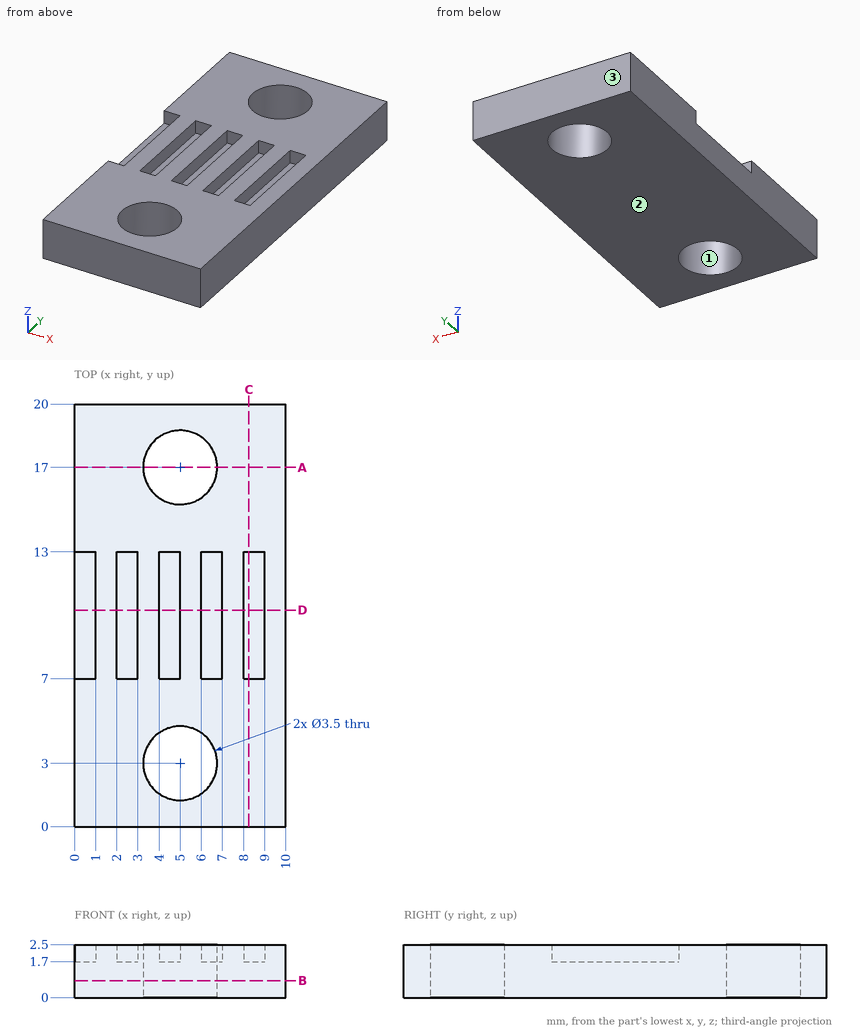
Answer from the drawing. Dimensions are ordinates in mm from the lowest x, y and z of the part. Give positions to 0.01 mm unless a question says otherwise; leave off trailing zeros. Order: outer loops, then holes, each group sorted by start corner. A loop starts at its lowest first (then second) coordinate and runs counter-clockwise, first axis right, second up. Notation, with made-up numbers: (-33, 53.25) -> (26, 53.25) arc R22 ccw to (26, 65.25) -> close; hole circle Ø6 at (49.5, -26). An arc over 180 degrees is marked (long way). Answer as a JSON object with one key per item and string values. Group by question number.
1. A flat-ended cylindrical pin translates along its axis: pin 1 Ø0.9 at (y, z) = (11, 2) entering from -X. Find the tip coordinate at first contact, or state that the pin passes through.
2. Section D-D on y = 10.25 is taken. Determine the outline of the cut face in (x, z), plus the area to 3 significant figures.
3. Section B-B on z = 0.8 is taken. Determine the outline of the cut face in (x, y).
4. Consider line 1 along X through (y, z) = (8.25, 1.75); line 2 along Y through (x, z) = (5, 1.1); line 3 along Y through (x, z) = (6.5, 1.55). Determine where each line is inside the solid, lowest interval first. Write a range as [from, to].
5. Section C-C on x = 8.25 is taken. Determine the outline of the cut face in (y, z).
6. The mould has two halves that part along Y. Classify the marked faces 1, 2 and 3: released by +Y, released by -Y, zero draft, split by the parting line, or undercut.
7. Section A-A on y = 17 is taken. Determine the outline of the cut face in (x, z).
Result sheet:
{
 "1": {"pin 1": "stops at x = 0"},
 "2": {"outline": "(0, 0) -> (10, 0) -> (10, 2.5) -> (9, 2.5) -> (9, 1.7) -> (8, 1.7) -> (8, 2.5) -> (7, 2.5) -> (7, 1.7) -> (6, 1.7) -> (6, 2.5) -> (5, 2.5) -> (5, 1.7) -> (4, 1.7) -> (4, 2.5) -> (3, 2.5) -> (3, 1.7) -> (2, 1.7) -> (2, 2.5) -> (1, 2.5) -> (1, 1.7) -> (0, 1.7) -> close", "area": "21.0 mm^2"},
 "3": {"outline": "(0, 0) -> (10, 0) -> (10, 20) -> (0, 20) -> close; hole circle Ø3.5 at (5, 3); hole circle Ø3.5 at (5, 17)"},
 "4": {"line 1": "x = [1, 2], [3, 4], [5, 6], [7, 8], [9, 10]", "line 2": "y = [0, 1.25], [4.75, 15.25], [18.75, 20]", "line 3": "y = [0, 2.1], [3.9, 16.1], [17.9, 20]"},
 "5": {"outline": "(0, 0) -> (20, 0) -> (20, 2.5) -> (13, 2.5) -> (13, 1.7) -> (7, 1.7) -> (7, 2.5) -> (0, 2.5) -> close"},
 "6": {"face 1": "undercut", "face 2": "zero draft", "face 3": "released by +Y"},
 "7": {"outline": "(0, 0) -> (3.25, 0) -> (3.25, 2.5) -> (0, 2.5) -> close; (6.75, 0) -> (10, 0) -> (10, 2.5) -> (6.75, 2.5) -> close"}
}
